Geometry: final body of the model. Coordinates: model frame, mm. Give positions to 0.01 mm unless a question says otherwise; leave off trailing zeros. Order: outer loops, then holes, each group sorted by start corner. A loop starts at its lowest first (then second) coordinate and runs counter-clockwise, first axis right, second up. Notation, with made-up numbers: (50, 26) -> (104, 26) arc R25 ccw to (104, 61) -> close; hole circle Ø5 at (-19.5, 11). An arc over 180 degrees is marked (long way). Write item = value, one per line.
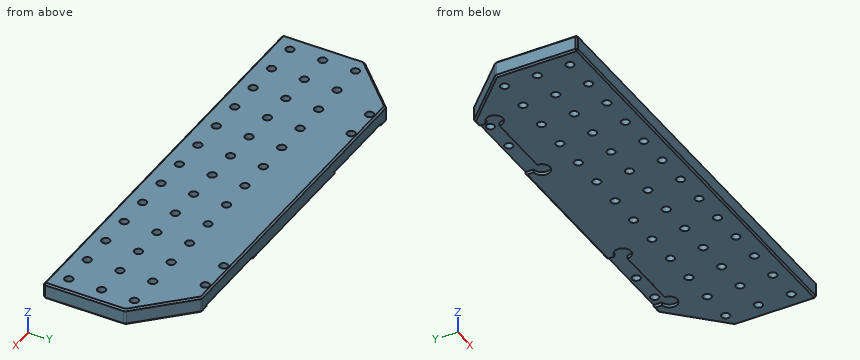
```python
from build123d import *

# Parameters (mm, degrees)
EXTRUDE_1_DEPTH             = 4
EXTRUDE_1_DEPTH_BACK        = 1
SKETCH_2_W                  = 130
SKETCH_2_H                  = 40
SKETCH_6_W                  = 25.606106999
SKETCH_6_H                  = 5
CUT_EXTRUDE_6_DEPTH         = 1
SKETCH_7_R                  = 2.5
CUT_EXTRUDE_7_DEPTH         = 1
CHAMFER_1_SIZE              = 15
M3X0_5_1_D                  = 2.5
FILLET_1_R                  = 1
M3X0_5_2_D                  = 2.5
PATTERN_LINEAR_1_COUNT      = 7
PATTERN_LINEAR_1_PITCH      = 10
PATTERN_LINEAR_1_COUNT_DIR2 = 3
PATTERN_LINEAR_1_PITCH_DIR2 = 10
PATTERN_LINEAR_2_COUNT      = 7
PATTERN_LINEAR_2_PITCH      = 10
PATTERN_LINEAR_2_COUNT_DIR2 = 3
PATTERN_LINEAR_2_PITCH_DIR2 = 10
CHAMFER_2_SIZE              = 0.5


with BuildPart() as part:
    # Sketch 2 → Extrude 1 (new, two sides: drawn at the far end of the back side and taken through both)
    with BuildSketch(Plane.XY.offset(-EXTRUDE_1_DEPTH_BACK)):
        with Locations((-80.49999999, -32)):
            Rectangle(SKETCH_2_W, SKETCH_2_H)
    extrude(amount=EXTRUDE_1_DEPTH + EXTRUDE_1_DEPTH_BACK)

    # Sketch 6 → Cut-Extrude 6 (cut)
    with BuildSketch(Plane(origin=(0, 0, -1), x_dir=(-1, 0, 0), z_dir=(0, 0, -1))):
        with Locations((115.285099269, -14.5)):
            Rectangle(SKETCH_6_W, SKETCH_6_H)
        with Locations((45.714900713, -14.5)):
            Rectangle(SKETCH_6_W, SKETCH_6_H)
    extrude(amount=-CUT_EXTRUDE_6_DEPTH, mode=Mode.SUBTRACT)

    # Sketch 7 → Cut-Extrude 7 (cut)
    with BuildSketch(Plane(origin=(0, 0, -1), x_dir=(-1, 0, 0), z_dir=(0, 0, -1))):
        with Locations((33.318100992, -17)):
            Circle(SKETCH_7_R)
        with Locations((128.088152768, -17)):
            Circle(SKETCH_7_R)
        with Locations((102.482045769, -17)):
            Circle(SKETCH_7_R)
        with Locations((58.517954212, -17)):
            Circle(SKETCH_7_R)
    extrude(amount=-CUT_EXTRUDE_7_DEPTH, mode=Mode.SUBTRACT)

    # Chamfer 1
    chamfer_1_edges = [part.edges().sort_by_distance(p)[0] for p in [
        (-145.49999999, -12, 1.5),
        (-15.49999999, -12, 1.5),
    ]]
    chamfer(chamfer_1_edges, length=CHAMFER_1_SIZE)

    # M3x0.5 _1 (through all)
    with Locations(Plane(origin=(0, 0, 0), x_dir=(-1, 0, 0), z_dir=(0, 0, -1))):
        with Locations((35.911847213, -14), (125.088152768, -14), (45.911847213, -14), (115.088152768, -14)):
            Hole(M3X0_5_1_D / 2)

    # Fillet 1
    fillet_1_edges = [part.edges().sort_by_distance(p)[0] for p in [
        (-30.49999999, -12, 1.5),
        (-130.49999999, -12, 1.5),
        (-145.49999999, -27, 1.5),
        (-15.49999999, -27, 1.5),
    ]]
    fillet(fillet_1_edges, radius=FILLET_1_R)

    # M3x0.5 _2 (through all)
    with Locations(Plane(origin=(0, 0, -1), x_dir=(-1, 0, 0), z_dir=(0, 0, -1))):
        with Locations((80.49999999, -47)):
            m3x0_5_2 = Hole(M3X0_5_2_D / 2)

    # Pattern Linear 1: M3x0.5 _2 7 × 3
    with Locations(*[(i * PATTERN_LINEAR_1_PITCH, j * PATTERN_LINEAR_1_PITCH_DIR2, 0) for i in range(PATTERN_LINEAR_1_COUNT) for j in range(PATTERN_LINEAR_1_COUNT_DIR2) if (i, j) != (0, 0)]):
        add(m3x0_5_2, mode=Mode.SUBTRACT)

    # Pattern Linear 2: M3x0.5 _2 7 × 3
    with Locations(*[(-i * PATTERN_LINEAR_2_PITCH, j * PATTERN_LINEAR_2_PITCH_DIR2, 0) for i in range(PATTERN_LINEAR_2_COUNT) for j in range(PATTERN_LINEAR_2_COUNT_DIR2) if (i, j) != (0, 0)]):
        add(m3x0_5_2, mode=Mode.SUBTRACT)

    # Chamfer 2
    chamfer_2_edges = [part.edges().sort_by_distance(p)[0] for p in [
        (-15.49999999, -39.707106781, -1),
        (-80.49999999, -52, 4),
        (-145.49999999, -39.707106781, 4),
        (-145.49999999, -39.707106781, -1),
        (-15.49999999, -39.707106781, 4),
        (-137.99999999, -19.5, -1),
        (-31.913030383, -12, -1),
        (-22.99999999, -19.5, -1),
        (-15.576120458, -27.03153013, -1),
        (-30.53153012, -12.076120467, -1),
        (-130.46846986, -12.076120467, -1),
        (-145.423879523, -27.03153013, -1),
        (-137.99999999, -19.5, 4),
        (-80.49999999, -12, 4),
        (-22.99999999, -19.5, 4),
        (-15.576120458, -27.03153013, 4),
        (-30.53153012, -12.076120467, 4),
        (-130.46846986, -12.076120467, 4),
        (-145.423879523, -27.03153013, 4),
        (-80.49999999, -12, -1),
        (-129.086969598, -12, -1),
        (-80.49999999, -52, -1),
        (-15.49999999, -52, 1.5),
        (-145.49999999, -52, 1.5),
    ]]
    chamfer(chamfer_2_edges, length=CHAMFER_2_SIZE)


solid = part.part
```
1) Section query C-C (x = -117.5). Output: boundary loops of the cut face in (y, z), plus the area to 3 significant figures.
Check sheet entries:
outline = (-52, -0.5) -> (-51.5, -1) -> (-17, -1) -> (-17, 0) -> (-12, 0) -> (-12, 3.5) -> (-12.5, 4) -> (-51.5, 4) -> (-52, 3.5) -> close
area = 195 mm²
2) Section query B-B (y = -47). Count the separate pieces of the cut face and the enclosed holes in it, plus the area to 3 significant figures.
Check sheet entries:
separate_pieces = 14
enclosed_holes = 0
area = 487 mm²
3) Line query: line 1 (Y direction, x = -110.5, z = 1.05); line 2 (Y direction, x = -45.5, z = 2.8); line 3 (Y direction, x = -52, z = -0.4). Output: solid intervals per line, ascending. Write a range as from..to.
Check sheet entries:
line_1 = -52..-48.25, -45.75..-38.25, -35.75..-28.25, -25.75..-12
line_2 = -52..-15.18, -12.82..-12
line_3 = -52..-17
4) Section query A-A (x = -50.5). Output: boundary loops of the cut face in (y, z).
Check sheet entries:
outline = (-52, -0.5) -> (-51.5, -1) -> (-48.25, -1) -> (-48.25, 4) -> (-51.5, 4) -> (-52, 3.5) -> close; (-45.75, -1) -> (-38.25, -1) -> (-38.25, 4) -> (-45.75, 4) -> close; (-35.75, -1) -> (-28.25, -1) -> (-28.25, 4) -> (-35.75, 4) -> close; (-25.75, -1) -> (-17, -1) -> (-17, 0) -> (-12, 0) -> (-12, 3.5) -> (-12.5, 4) -> (-25.75, 4) -> close
5) First-contact query: P1, Ø1.5, axis at x = -60.5, y = -47, coming from the +Z side; P2, Ø4, axis at x = -70.5, y = -27, coming from the +Z side; P3, Ø1.5, axis at y = -20.5, z = 1.5, coming from the +X side; P4, Ø0.5, axis at y = -13.5, z = -0.5, coming from the +X side. Flat tips, straight axial feed; report the tip coordinate or a pass-through.
Check sheet entries:
P1 = through
P2 = 4
P3 = -21.25
P4 = -28.75
